CAD build for the part. Positions are in the model's coordinates, mm. Face numbers are marked on the shaded views. Give positions to 0.01 mm unless a question says otherwise; leave off trailing zeros. Loops run counter-clockwise (first coordinate to the right, second up) from the corner with the lowest first, then second, coordinate; pieces in that order, holes last. Notation, with made-up numbers: (-28.5, 1) - (-3.5, 1) arc R26 cw to (-3.5, 33) - close; hole circle Ø10 at (29.25, -5.75). An arc over 180 degrees is marked (long way). Return JSON: item names as keys, results as strings.
Autodesk Inventor part; units mm, degrees
ref_plane "YZ Plane" through (0, 0, 0) normal (1, 0, 0) x (0, 1, 0)
ref_plane "XZ Plane" through (0, 0, 0) normal (0, 1, 0) x (-1, 0, 0)
ref_plane "XY Plane" through (0, 0, 0) normal (0, 0, 1) x (1, 0, 0)
sketch "Sketch1" plane through (0, 0, 0) normal (0, 0, 1) x (1, 0, 0)
  circle A0 centre (-43.9941, 0) radius 9.525
  circle A1 centre (43.9941, 0) radius 6.35
  line L0 (43.9941, 0) -> (-43.9941, 0) construction
  line L1 (43.9941, 12.7) -> (-43.9941, 12.7)
  line L2 (-43.9941, -12.7) -> (43.9941, -12.7)
  arc A2 (43.9941, -12.7) -> (43.9941, 12.7) centre (43.9941, 0) ccw
  arc A3 (-43.9941, 12.7) -> (-43.9941, -12.7) centre (-43.9941, 0) ccw
  point P0 (0, 0)
  point P1 (0, 0)
  dimension "d10" = 12.7
  dimension "d11" = 19.05
  dimension "d12" = 87.9881
  dimension "d13" = 12.7
extrude "Extrusion1" add sketch "Sketch1" against normal blind 12.7
extrude "Extrusion2" add sketch "Sketch1" along normal blind 31.6653 and the other way blind 12.7 contours A0
sketch "Sketch2" plane through (0, 0, 0) normal (0, 0, 1) x (1, 0, 0)
  circle A0 centre (-43.9941, 0) radius 9.525
  circle A1 centre (-43.9941, 0) radius 10.033
  point P0 (0, 0)
  dimension "d20" = 20.066
extrude "Extrusion3" add sketch "Sketch2" along normal blind 1
properties part number "Frame"
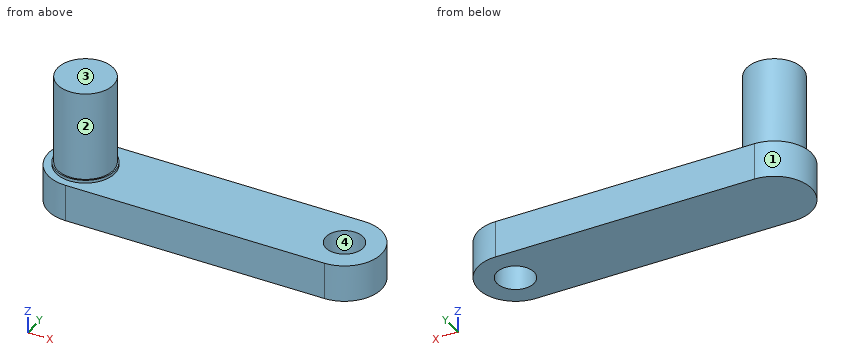
1. Cut at C-C, the plane x = -39.5. Write the cut outline in (y, z), plus the area to 3 significant figures.
Values follow:
{"outline": "(-12.7, -12.7) - (12.7, -12.7) - (12.7, 0) - (8.97, 0) - (8.97, 1) - (8.4, 1) - (8.4, 31.67) - (-8.4, 31.67) - (-8.4, 1) - (-8.97, 1) - (-8.97, 0) - (-12.7, 0) - close", "area": "856 mm²"}
2. Drop flat-ended pins along their axis: P1, Ø2, axis at y = -1, z = 25.5, coming from the +X side; P2, Ø6, axis at y = 4, z = -2, coming from the -X side; P3, Ø7.5, axis at x = 23, y = -3, coming from the +Z side. Give the stop position or say it passes through.
Values follow:
{"P1": "stops at x = -34.47", "P2": "stops at x = -56.65", "P3": "stops at z = 0"}
3. Pull direction X, two halves, no side cores. Call the marked faces 1, 2, 3 and 4: +X half, -X half, draft (parallel to the pull), parting line (faces both ways), or undercut.
Values follow:
{"face 1": "-X half", "face 2": "parting line", "face 3": "draft", "face 4": "undercut"}
4. Cut at D-D, the plane y = -8. Write the cut outline in (x, z).
Values follow:
{"outline": "(-53.86, -12.7) - (53.86, -12.7) - (53.86, 0) - (-37.94, 0) - (-37.94, 1) - (-38.82, 1) - (-38.82, 31.67) - (-49.16, 31.67) - (-49.16, 1) - (-50.05, 1) - (-50.05, 0) - (-53.86, 0) - close"}
5. Drill centre lines: probe 1 along Z at (x, y) = (25, 3); probe 2 along X at (y, z) = (-0.25, -9); probe 3 along X at (y, z) = (-4.75, -8). Where is each one in solid material? Low to high.
Values follow:
{"probe 1": "z = -12.7 to 0", "probe 2": "x = -56.69 to 37.65, 50.34 to 56.69", "probe 3": "x = -55.77 to 39.78, 48.21 to 55.77"}
6. Cut at B-B, the plane z = -7.5. Write the cut outline in (x, y), plus the area to 3 significant figures.
Values follow:
{"outline": "(-43.99, -12.7) - (43.99, -12.7) arc R12.7 ccw to (43.99, 12.7) - (-43.99, 12.7) arc R12.7 ccw to start; hole circle Ø12.7 at (43.99, 0)", "area": "2,610 mm²"}
7. Cut at A-A, the plane y = 0. Write the cut outline in (x, z), plus the area to 3 significant figures.
Values follow:
{"outline": "(-56.69, -12.7) - (37.64, -12.7) - (37.64, 0) - (-33.96, 0) - (-33.96, 1) - (-34.47, 1) - (-34.47, 31.67) - (-53.52, 31.67) - (-53.52, 1) - (-54.03, 1) - (-54.03, 0) - (-56.69, 0) - close; (50.34, -12.7) - (56.69, -12.7) - (56.69, 0) - (50.34, 0) - close", "area": "1,880 mm²"}
